Part model, mm, in its own coordinate system. Face numbers are marked on the shaded views. Coordinates: 2 decimals unless noted, no trailing zeros. Loops run counter-clockwise (first coordinate to the right, second up) from the corner with the lowest first, then second, coordinate; pieces in that order, holes last. Notation, with made-up numbers: M 24,58 L 52,58 A19 cw 52,86 Z; hole C 15,28.25 d8. An arc over 180 degrees is marked long. Use a Markdown table: item, result. Add a question column.
1) Pull direction X, two halves, no side cores. Call the marked faces 1, 2 and 3: released by +X, released by -X, zero draft, split by the parting line, or undercut.
2) Band-saw the part on D-D (x = -16). List the corners of the cut face in (y, z).
3) Band-saw the part on A-A (y = 0). List the corners of the cut face in (x, z).
4) Band-saw the part on B-B (z = 0). List the corners of the cut face in (x, y), plus the area to 3 significant figures.
5) Wall check: probe 1 along X at (y, z) = (0, 1); probe 2 along Y at (x, z) = (-16.5, -1.25); probe 3 along Y at (x, z) = (-16.5, 2). Give the ranges that are in metal, low to high. Write a range as from..to.
6) Pin check, flat tips, straight feed: pin 1 Ø6 at (x, z) = (-3.5, -2.5) entering from +Y; pin 2 Ø4 at (x, z) = (-17, 3.5) entering from +Y; pin 3 Ø1.5 at (x, y) = (-11.5, -3) entering from -Z; pin 4 Ø1 at (x, y) = (-4.5, -2) entering from +Z. Stop position of each tip, or through.
7) Band-saw the part on C-C (x = -4). List the corners of the cut face in (y, z).
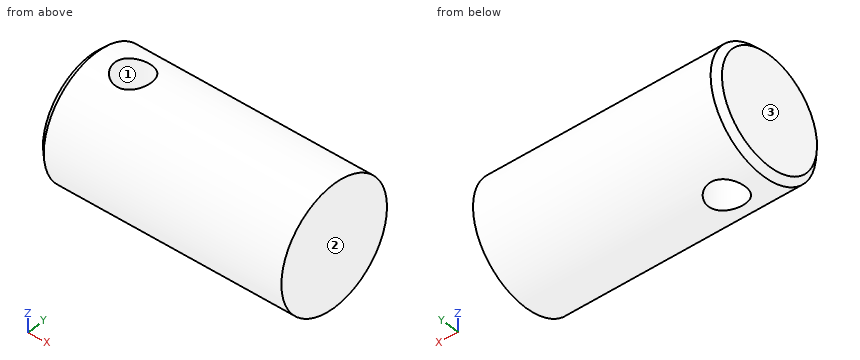
from build123d import *

# Parameters (mm, degrees)
ESQUISSE1_W           = 20
ESQUISSE1_H           = 5
CHANFREIN1_SIZE       = 0.5
EXTRUSION1_DEPTH      = 22.213203436
EXTRUSION1_DEPTH_BACK = 22.213203436
ESQUISSE2_R           = 1.5


with BuildPart() as part:
    # Esquisse1 → Base-Révolution (revolve)
    with BuildSketch(Plane.XY, mode=Mode.PRIVATE) as base_r_volution_sk:
        with Locations((-10, 2.5)):
            Rectangle(ESQUISSE1_W, ESQUISSE1_H)
    revolve(base_r_volution_sk.sketch.rotate(Axis((0, 0, 0), (-1, 0, 0)), 90), axis=Axis((0, 0, 0), (-1, 0, 0)))

    # Chanfrein1
    chanfrein1_edges = [part.edges().sort_by_distance(p)[0] for p in [
        (-20, 0, 5),
    ]]
    chamfer(chanfrein1_edges, length=CHANFREIN1_SIZE)

    # Esquisse2 → Extrusion1 (cut, two sides: drawn at the far end of the back side and taken through both)
    with BuildSketch(Plane.XY.offset(-EXTRUSION1_DEPTH_BACK)):
        with Locations((-16.5, 0)):
            Circle(ESQUISSE2_R)
    extrude(amount=EXTRUSION1_DEPTH + EXTRUSION1_DEPTH_BACK, mode=Mode.SUBTRACT)


solid = part.part
Entries:
| question | item | result |
|---|---|---|
| 1 | face 1 | undercut |
| 1 | face 2 | released by +X |
| 1 | face 3 | released by -X |
| 2 | outline | M -1.41,-4.8 L -1.41,4.8 A5 ccw Z; M 1.41,-4.8 A5 ccw 1.41,4.8 Z |
| 3 | outline | M -20,-4.5 L -19.5,-5 L -18,-5 L -18,5 L -19.5,5 L -20,4.5 Z; M -15,-5 L 0,-5 L 0,5 L -15,5 Z |
| 4 | outline | M -20,-4.5 L -19.5,-5 L 0,-5 L 0,5 L -19.5,5 L -20,4.5 Z; hole C -16.5,0 d3 |
| 4 | area | 193 mm2 |
| 5 | probe 1 | -20..-18, -15..0 |
| 5 | probe 2 | -4.84..-1.5, 1.5..4.84 |
| 5 | probe 3 | -4.58..-1.5, 1.5..4.58 |
| 6 | pin 1 | y = 5 |
| 6 | pin 2 | y = 4.77 |
| 6 | pin 3 | z = -4.47 |
| 6 | pin 4 | z = 4.77 |
| 7 | outline | C 0,0 d10 |
